Verification items for the finished model (mm, model axes). Face numbers are marked on the shaded views. A direction names the side the tool comes from. Give positions to 0.01 mm unless a question says otherwise; leave off trailing zeros. Write each loop counter-clockwise with the first axis right and the second up, starting at its lowest first coordinate (ties: lowest second). Pieces come first, ordered by that corner, then holes. Notation, with made-up numbers: (65, -26) -> (120, -26) arc R10 cw to (120, -16) -> close; hole circle Ø1 at (13, 2.25). An arc over 180 degrees is marked (long way). Answer as CSV lines item,"result". Start each with the question number.
1) Gauge pin test, flat ends, axial feed: pin 1 Ø1 at (y, z) = (-46, -40.5) entering from -X; pin 2 Ø2 at (x, z) = (15, 48) entering from -Y; pin 3 Ø1.5 at (x, z) = (-4.5, -23) entering from +Y. Record the tip position at first contact, or that the pin passes through.
2) Tool access check on the marked faces 5 and 6. Record the directions out of +Z, -Z, +X, -X, +Y, -Y that give a thin tool (end or side, any length) a straight path to the whole face; none if there is none.
3) Material ranges on L1, parallel to Z at x = 22, y = -5; L2, parallel to Z at x = 14.5, y = -3.5; L3, parallel to Z at x = 15, y = 34, recorded low to high.
4) Sectioned sample at B-B on z = 45. Record the cut outline in (x, y), and give its area (3 significant figures).
5) Mould release check, pull along Z, two halves, no side actions. Record for the marked faces 1, 2, 3 and 4: released by +Z, released by -Z, zero draft, split by the parting line, or undercut.
6) Sectioned sample at A-A on y = 0. Record the cut outline in (x, z), and give its area (3 significant figures).
7) Sectioned sample at D-D on x = 18.5. Give the number of separate pieces and of enclosed holes in the cut face, and give its area (3 significant figures).
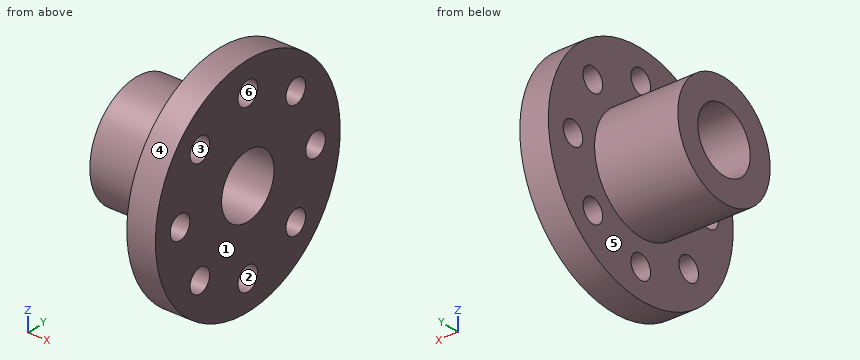
```python
from build123d import *

# Parameters (mm, degrees)
F2_R     = 6.5
F3_DEPTH = 15.567862


with BuildPart() as f1:
    # F0 (on Front) → F1 (revolve)
    with BuildSketch(Plane.XZ):
        Polygon((-36.170062, 17.398257), (24.723839, 17.398257), (24.723839, 61.351746), (9.156977, 61.351746), (9.156977, 30.675873), (-36.170062, 30.675873), align=None)
    revolve(axis=Axis((-16.482558, 0, 0), (-1, 0, 0)))

    # F2 (on face) → F3 (cut, through all)
    with BuildSketch(Plane(origin=(9.156977, 0, 0), x_dir=(0, -1, 0), z_dir=(-1, 0, 0))):
        with Locations((0, 45)):
            Circle(F2_R)
        with Locations((-31.819805, 31.819805)):
            Circle(F2_R)
        with Locations((-45, 0)):
            Circle(F2_R)
        with Locations((-31.819805, -31.819805)):
            Circle(F2_R)
        with Locations((0, -45)):
            Circle(F2_R)
        with Locations((31.819805, -31.819805)):
            Circle(F2_R)
        with Locations((45, 0)):
            Circle(F2_R)
        with Locations((31.819805, 31.819805)):
            Circle(F2_R)
    extrude(amount=-F3_DEPTH, mode=Mode.SUBTRACT)


solid = f1.part
```
Ans:
1,pin 1,"stops at x = 9.16"
1,pin 2,"stops at y = -39.43"
1,pin 3,"stops at y = 21.12"
2,face 5,"-X"
2,face 6,"+X, -X"
3,L1,"z = -61.15 to -49.15, -40.85 to -16.66, 16.66 to 40.85, 49.15 to 61.15"
3,L2,"z = -61.25 to -50.48, -39.52 to -17.04, 17.04 to 39.52, 50.48 to 61.25"
3,L3,"z = -51.07 to -37.94, -25.7 to 25.7, 37.94 to 51.07"
4,outline,"(9.16, -41.7) -> (24.72, -41.7) -> (24.72, -6.5) -> (9.16, -6.5) -> close; (9.16, 6.5) -> (24.72, 6.5) -> (24.72, 41.7) -> (9.16, 41.7) -> close"
4,area,"1,100 mm²"
5,face 1,"zero draft"
5,face 2,"undercut"
5,face 3,"undercut"
5,face 4,"split by the parting line"
6,outline,"(-36.17, -30.68) -> (9.16, -30.68) -> (9.16, -38.5) -> (24.72, -38.5) -> (24.72, -17.4) -> (-36.17, -17.4) -> close; (-36.17, 17.4) -> (24.72, 17.4) -> (24.72, 38.5) -> (9.16, 38.5) -> (9.16, 30.68) -> (-36.17, 30.68) -> close; (9.16, -61.35) -> (24.72, -61.35) -> (24.72, -51.5) -> (9.16, -51.5) -> close; (9.16, 51.5) -> (24.72, 51.5) -> (24.72, 61.35) -> (9.16, 61.35) -> close"
6,area,"2,170 mm²"
7,separate pieces,"1"
7,enclosed holes,"9"
7,area,"9,810 mm²"
